For this review, take the finished solid that the model builds, in its own axes (mm). Coordinates: 2 decimals unless noted, no trailing zeros. Loops run counter-clockwise (first coordinate to the right, second up) from the corner with the lowest first, then second, coordinate; pieces in that order, holes last. Notation, with made-up numbers: (47.5, 47.5) - (56.5, 47.5) arc R14 cw to (56.5, 71.5) - close; hole circle Ø8 at (-6.75, -25.5). An arc over 180 degrees is marked (long way). One line per item, written item: value. Start each with the question number.
1. Take a section at A-A, the plane y = 70. State the section outline as (x, z) points.
2. Take a section at B-B, the plane x = 30. State the section outline as (y, z) points.
3. Insertion check: pin 1 (8 mm diameter, centred on y = 70, z = 62.5, fed in from -X); pin 2 (12 mm diameter, centred on x = 91, y = 78, fed in from +Z). Each pin has a flat end and moves straight along its axis. Give the tip position at first contact, or say it passes through.
4. Take a section at D-D, the plane y = 17. State the section outline as (x, z) points.
5. Take a section at C-C, the plane z = 33. State the section outline as (x, y) points.
6. To check wall thickness, follow line 1 (Z direction, x = 68, y = 73.5); line 2 (Y direction, x = 30, z = 56); line 3 (X direction, y = 81.5, z = 40). State the ranges of each line that lie inside material, in increasing order. Write a range as from..to.
```python
from build123d import *

# Parameters (mm, degrees)
CROQUIS1_W              = 120
CROQUIS1_H              = 100
SALIENTE_EXTRUIR1_DEPTH = 30
CROQUIS3_R              = 15
SALIENTE_EXTRUIR3_DEPTH = 40
SALIENTE_EXTRUIR3_TAPER = 4


with BuildPart() as part:
    # Croquis1 → Saliente-Extruir1 (new body)
    with BuildSketch(Plane.XY):
        with Locations((60, 50)):
            Rectangle(CROQUIS1_W, CROQUIS1_H)
    extrude(amount=SALIENTE_EXTRUIR1_DEPTH)

    # Croquis3 → Saliente-Extruir3 (add)
    with BuildSketch(Plane.XY.offset(30)):
        with Locations((30, 70)):
            Circle(CROQUIS3_R)
    extrude(amount=SALIENTE_EXTRUIR3_DEPTH, taper=SALIENTE_EXTRUIR3_TAPER)


solid = part.part
```
Solutions:
1. outline: (0, 0) - (120, 0) - (120, 30) - (45, 30) - (42.2, 70) - (17.8, 70) - (15, 30) - (0, 30) - close
2. outline: (0, 0) - (100, 0) - (100, 30) - (85, 30) - (82.2, 70) - (57.8, 70) - (55, 30) - (0, 30) - close
3. pin 1: x = 16.99
3. pin 2: z = 30
4. outline: (0, 0) - (120, 0) - (120, 30) - (0, 30) - close
5. outline: circle Ø29.58 at (30, 70)
6. line 1: 0..30
6. line 2: 56.82..83.18
6. line 3: 21.5..38.5
